from build123d import *

# Parameters (mm, degrees)
BOSS_EXTRUDE1_DEPTH = 18.25625


with BuildPart() as part:
    # Sketch1 → Boss-Extrude1 (new body)
    with BuildSketch(Plane.XY):
        with BuildLine():
            ThreePointArc((-368.315070695, 1468.660053657), (-1109.186200683, 1161.781183645), (-1416.065070695, 420.910053657))
            Line((-1416.065070695, 420.910053657), (-1416.065070695, -188.062492737))
            Line((-1416.065070695, -188.062492737), (-1358.915070695, -188.062492737))
            Line((-1358.915070695, -188.062492737), (-1358.915070695, -48.362492737))
            Line((-1358.915070695, -48.362492737), (-1320.815070695, -48.362492737))
            Line((-1320.815070695, -48.362492737), (-1320.815070695, -188.062492737))
            Line((-1320.815070695, -188.062492737), (-1263.665070695, -188.062492737))
            Line((-1263.665070695, -188.062492737), (-1263.665070695, 420.910053657))
            ThreePointArc((-1263.665070695, 420.910053657), (-1001.42312723, 1054.018110192), (-368.315070695, 1316.260053657))
            Line((-368.315070695, 1316.260053657), (-368.315070695, 1468.660053657))
        make_face()
    extrude(amount=BOSS_EXTRUDE1_DEPTH)


solid = part.part
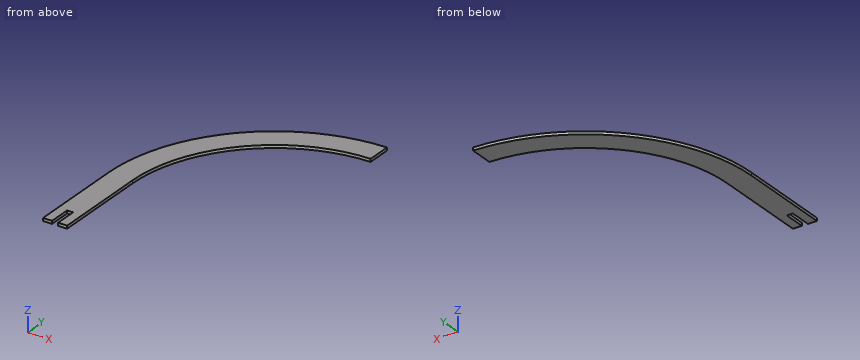
Input: part model. Units: mm. Frame: model coordinates. Round coordinates to 2 decimals unless told otherwise and drop trailing zeros. Order: outer loops, then holes, each group sorted by start corner. A loop starts at its lowest first (then second) coordinate and runs counter-clockwise, first axis right, second up.
1. Pin query (flat end, axial travel): P1, Ø3, axis at y = 1054, z = 13.5, coming from the +X side; P2, Ø1, axis at y = 978.5, z = 12, coming from the -X side; P3, Ø9, axis at y = -143, z = 5, coming from the +X side. Return the tip coordinate at first contact, or that it passes through.
The answers:
P1: stops at x = -999.94
P2: stops at x = -1255.69
P3: stops at x = -1263.67
2. Cut plane B-B, the plane y = 353. Output: boundary loops of the cut face in (x, z).
The answers:
outline: (-1416.07, 0) - (-1263.67, 0) - (-1263.67, 18.26) - (-1416.07, 18.26) - close
3. Cut plane C-C, the plane x = -480. Output: boundary loops of the cut face in (y, z).
The answers:
outline: (1309.27, 0) - (1462.69, 0) - (1462.69, 18.26) - (1309.27, 18.26) - close
4. Material intervals for line 1 (X direction, y = 290, z = 7); line 2 (Y direction, x = -918, z = 14.5); line 3 (X direction, y = 1132.5, z = 1), sorted ascending.
The answers:
line 1: x = -1416.07 to -1263.67
line 2: y = 1127.66 to 1312.89
line 3: x = -1137.35 to -911.72
5. Cut plane A-A, the plane z = 13.25. Output: boundary loops of the cut face in (x, y), then the cut area to 3 significant figures.
The answers:
outline: (-1416.07, -188.06) - (-1358.92, -188.06) - (-1358.92, -48.36) - (-1320.82, -48.36) - (-1320.82, -188.06) - (-1263.67, -188.06) - (-1263.67, 420.91) arc R895.35 cw to (-368.32, 1316.26) - (-368.32, 1468.66) arc R1047.75 ccw to (-1416.07, 420.91) - close
area: 320,000 mm2
